```python
from build123d import *

# Parameters (mm, degrees)
F0_W     = 600
F0_H     = 50
F1_DEPTH = 50
F2_R     = 5
F3_DEPTH = 50.001
F4_R     = 24.99999


# Not quite as in the source:
# - a fillet or chamfer is up to 0.001 mm smaller than in the source, because OpenCascade refuses the exact size


with BuildPart() as f1:
    # F0 (on Front) → F1 (new body)
    with BuildSketch(Plane.XZ):
        with Locations((0, 10.9999733963)):
            Rectangle(F0_W, F0_H)
    extrude(amount=F1_DEPTH)

    # F2 (on face) → F3 (cut, through all)
    with BuildSketch(Plane.XY.offset(35.9999733963)):
        with Locations((50, -25)):
            Circle(F2_R)
        with Locations((-200, -25)):
            Circle(F2_R)
        with Locations((100, -25)):
            Circle(F2_R)
        with Locations((-150, -24.9278768897)):
            Circle(F2_R)
    extrude(amount=-F3_DEPTH, mode=Mode.SUBTRACT)

    # F4 (radius 25 in the source; OpenCascade refuses exactly that, so slightly less here)
    f4_edges = [f1.edges().sort_by_distance(p)[0] for p in [
        (-300, 0, 10.999973),
        (-300, -50, 10.999973),
    ]]
    fillet(f4_edges, radius=F4_R)


solid = f1.part
```
Geometry: final body of the model. Coordinates: model frame, mm. Coordinates: 2 decimals unless noted, no trailing zeros. Write each loop counter-clockwise with the first axis right and the second up, starting at its lowest first coordinate (ties: lowest second). Pieces come first, ordered by that corner, then holes. Notation, with made-up numbers: M -6.75,44 L 40.25,44 A12 cw 40.25,58 Z; hole C 4,82.5 d1. An arc over 180 degrees is marked long. Answer as CSV lines item,"result". Start each with the question number.
Q1. Cut plane B-B on z = 14.5. Count the separate pieces of the cut face and the enclosed holes in it, then the cut area to 3 significant figures.
Q2. Mould query, pull axis Y, two halves, no side actions, for faces 1 (the cylindrical face through (-197.693, -29.436, 11.35)), 2 (the flat face through (-4, -25, 36)), 3 (the cylindrical face through (-292.871, -42.482, 11.35)). Classes: released by +Y, released by -Y, zero draft, split by the parting line, or undercut.
Q3. Cut plane A-A on x = -150. Return the cut outline in (y, z).
Q4. Line query: line 1 (Y direction, x = -150, z = 12.5); line 2 (Y direction, x = 100, z = 11.5); line 3 (X direction, y = -25.5, z = 7.5) (3 decimals). Output: solid intervals per line, ascending. Write a range as from..to.
Q5. Pin query (flat end, axial travel): P1, Ø1, axis at y = -18.5, z = -7.5, coming from the -X side. Return the tip coordinate at first contact, or that it passes through.
Findings below:
1,separate pieces,"1"
1,enclosed holes,"4"
1,area,"29,400 mm2"
2,face 1,"undercut"
2,face 2,"zero draft"
2,face 3,"released by -Y"
3,outline,"M -50,-14 L -29.93,-14 L -29.93,36 L -50,36 Z; M -19.93,-14 L 0,-14 L 0,36 L -19.93,36 Z"
4,line 1,"y = -50..-29.93, -19.93..0"
4,line 2,"y = -50..-30, -20..0"
4,line 3,"x = -299.995..-204.975, -195.025..-154.967, -145.033..45.025, 54.975..95.025, 104.975..300"
5,P1,"stops at x = -299.27"
